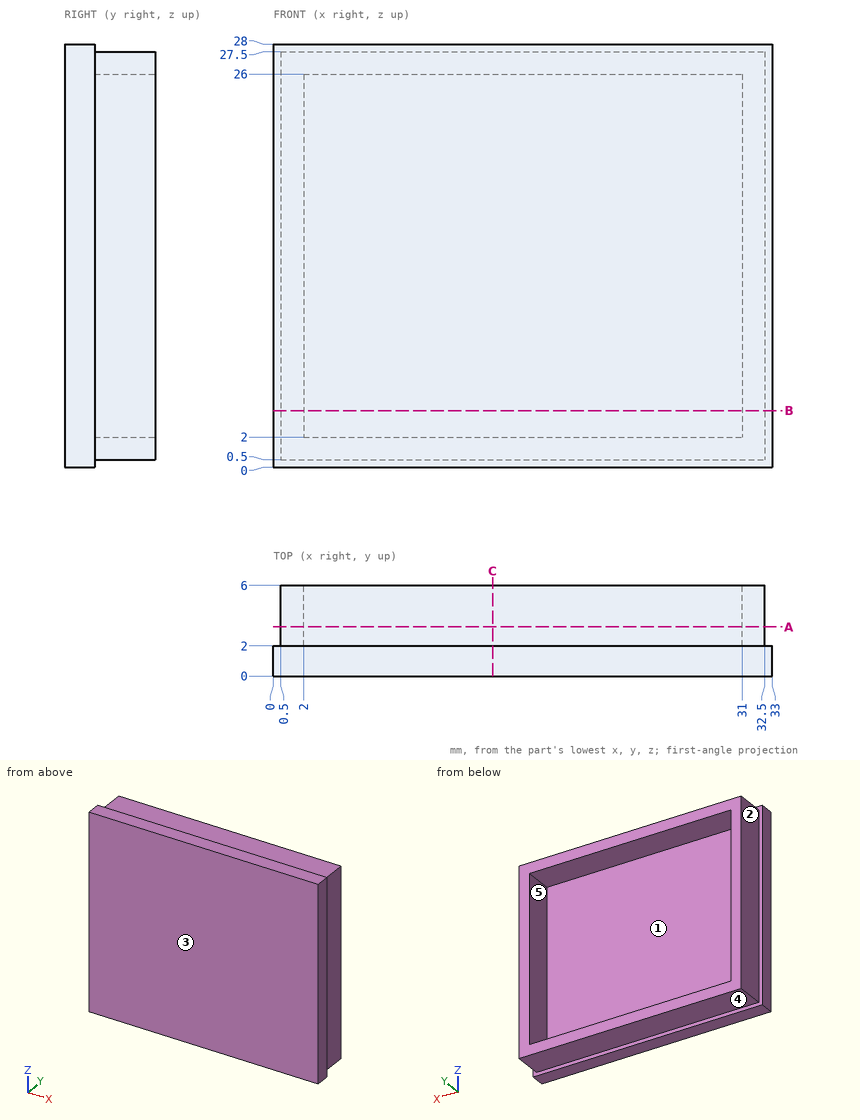
Check sheet for the drawn part. Datum: minimum x, y, z corner. Units: mm. A direction names the side the tool comes from. Coordinates: 2 decimals unless noted, no trailing zeros. Loops run counter-clockwise (first coordinate to the right, second up) from the corner with the lowest first, then second, coordinate; pieces in that order, holes last. Notation, with made-up numbers: (7, -30) -> (29, -30) arc R12 ccw to (29, -9) -> close; hole circle Ø11 at (83.25, 81.25). An arc over 180 degrees is marked (long way). Answer as CSV lines item,"result".
1) Cross-section at B-B, the plane z = 3.75. Record the cut outline in (x, y).
Found:
outline,"(0, 0) -> (33, 0) -> (33, 2) -> (32.5, 2) -> (32.5, 6) -> (31, 6) -> (31, 2) -> (2, 2) -> (2, 6) -> (0.5, 6) -> (0.5, 2) -> (0, 2) -> close"
2) Cross-section at A-A, the plane y = 3.25. Record the cut outline in (x, z).
Found:
outline,"(0.5, 0.5) -> (32.5, 0.5) -> (32.5, 27.5) -> (0.5, 27.5) -> close; hole (2, 2) -> (31, 2) -> (31, 26) -> (2, 26) -> close"
3) Depth check by flat-ended pin: pin 1 (1.2 mm diameter, centred on y = 5, z = 14.5, fed in from -X); pin 2 (2 mm diameter, centred on x = 16, z = 24, fed in from +Y); pin 3 (2 mm diameter, centred on x = 9.5, y = 4.5, fed in from +Z). Enter the tip coordinate at first touch or a pass-through.
Found:
pin 1,"stops at x = 0.5"
pin 2,"stops at y = 2"
pin 3,"stops at z = 27.5"
4) Release check for a two-part mould opening along Z. For the marked faces 3, 4 and 5 record: +Z half, -Z half, draft (parallel to the pull), parting line (faces both ways), or undercut.
Found:
face 3,"draft"
face 4,"-Z half"
face 5,"undercut"
5) Thickness scan on L1, parallel to X at y = 2.85, z = 11.5; L2, parallel to Z at x = 20, y = 3.95; L3, parallel to Y at x = 6, z = 3.75. Record the ranges inside material, lowest first. Write a range as from..to.
Found:
L1,"x = 0.5..2, 31..32.5"
L2,"z = 0.5..2, 26..27.5"
L3,"y = 0..2"
6) Tool access check on the marked faces 1 and 2. Record the directions out of +Z, -Z, +X, -X, +Y, -Y that give a thin tool (end or side, any length) a straight path to the whole face; none if there is none.
Found:
face 1,"+Y"
face 2,"+Z, -Z, -X, +Y"
7) Cross-section at C-C, the plane x = 14.5. Record the cut outline in (y, z), then the cut area to 3 significant figures.
Found:
outline,"(0, 0) -> (2, 0) -> (2, 0.5) -> (6, 0.5) -> (6, 2) -> (2, 2) -> (2, 26) -> (6, 26) -> (6, 27.5) -> (2, 27.5) -> (2, 28) -> (0, 28) -> close"
area,"68.0 mm2"
